```python
from build123d import *

# Parameters (mm, degrees)
SKETCH1_R                = 130.175
SKETCH1_R_2              = 7.874
EXTRUDE1_DEPTH           = 8.89
SKETCH3_R                = 38.1
EXTRUDE3_DEPTH           = 185.309775514
SKETCH4_R                = 5.588
EXTRUDE4_DEPTH           = 185.309775514
EXTRUDE9_DEPTH           = 185.309775514
FILLET1_R                = 7.62
FILLET2_R                = 10.16
CIRPATTERN1_COUNT        = 5
FILLET1_OF_CIRPATTERN1_R = 7.62
FILLET2_OF_CIRPATTERN1_R = 10.16


with BuildPart() as part:
    # Sketch1 → Extrude1 (new body)
    with BuildSketch(Plane.XY):
        Circle(SKETCH1_R)
        with Locations((0, 55)):
            Circle(SKETCH1_R_2, mode=Mode.SUBTRACT)
        with Locations((52.308108396, 16.995934691)):
            Circle(SKETCH1_R_2, mode=Mode.SUBTRACT)
        with Locations((32.328188876, -44.495934691)):
            Circle(SKETCH1_R_2, mode=Mode.SUBTRACT)
        with Locations((-32.328188876, -44.495934691)):
            Circle(SKETCH1_R_2, mode=Mode.SUBTRACT)
        with Locations((-52.308108396, 16.995934691)):
            Circle(SKETCH1_R_2, mode=Mode.SUBTRACT)
    extrude(amount=EXTRUDE1_DEPTH)

    # Sketch3 → Extrude3 (cut, through all)
    with BuildSketch(Plane(origin=(0, 0, 0), x_dir=(-1, 0, 0), z_dir=(0, 0, -1))):
        Circle(SKETCH3_R)
    extrude(amount=-EXTRUDE3_DEPTH, mode=Mode.SUBTRACT)

    # Sketch4 → Extrude4 (cut, through all)
    with BuildSketch(Plane.XY.offset(8.89)):
        with Locations((0, 114.3)):
            Circle(SKETCH4_R)
        with Locations((14.540907903, 100.554074991)):
            Circle(SKETCH4_R)
        with Locations((25.431391759, 85.18482443)):
            Circle(SKETCH4_R)
        with Locations((70.868043945, 72.803024301)):
            Circle(SKETCH4_R)
        with Locations((70.644811643, 53.967773605)):
            Circle(SKETCH4_R)
        with Locations((67.183854337, 92.470642457)):
            Circle(SKETCH4_R)
        with Locations((100.125995916, 17.243692812)):
            Circle(SKETCH4_R)
        with Locations((88.874314608, 2.13686756)):
            Circle(SKETCH4_R)
        with Locations((108.705759813, 35.320642457)):
            Circle(SKETCH4_R)
        with Locations((91.139220605, -44.90214324)):
            Circle(SKETCH4_R)
        with Locations((73.156850119, -50.510249263)):
            Circle(SKETCH4_R)
        with Locations((108.705759813, -35.320642457)):
            Circle(SKETCH4_R)
        with Locations((47.34036073, -89.896886742)):
            Circle(SKETCH4_R)
        with Locations((29.495955395, -83.864167648)):
            Circle(SKETCH4_R)
        with Locations((67.183854337, -92.470642457)):
            Circle(SKETCH4_R)
        with Locations((-14.540907903, -100.554074991)):
            Circle(SKETCH4_R)
        with Locations((-25.431391759, -85.18482443)):
            Circle(SKETCH4_R)
        with Locations((0, -114.3)):
            Circle(SKETCH4_R)
        with Locations((-70.868043945, -72.803024301)):
            Circle(SKETCH4_R)
        with Locations((-70.644811643, -53.967773605)):
            Circle(SKETCH4_R)
        with Locations((-67.183854337, -92.470642457)):
            Circle(SKETCH4_R)
        with Locations((-100.125995916, -17.243692812)):
            Circle(SKETCH4_R)
        with Locations((-88.874314608, -2.13686756)):
            Circle(SKETCH4_R)
        with Locations((-108.705759813, -35.320642457)):
            Circle(SKETCH4_R)
        with Locations((-91.139220605, 44.90214324)):
            Circle(SKETCH4_R)
        with Locations((-73.156850119, 50.510249263)):
            Circle(SKETCH4_R)
        with Locations((-108.705759813, 35.320642457)):
            Circle(SKETCH4_R)
        with Locations((-47.34036073, 89.896886742)):
            Circle(SKETCH4_R)
        with Locations((-29.495955395, 83.864167648)):
            Circle(SKETCH4_R)
        with Locations((-67.183854337, 92.470642457)):
            Circle(SKETCH4_R)
    extrude(amount=-EXTRUDE4_DEPTH, mode=Mode.SUBTRACT)

    # Sketch8 → Extrude9 (cut, through all)
    with BuildSketch(Plane.XY.offset(8.89)):
        Polygon((28.096692809, 71.081575805), (58.920240294, 48.686957693), (31.388364268, 21.595846559), (10.839332611, 36.525591967), align=None)
    extrude9 = extrude(amount=-EXTRUDE9_DEPTH, mode=Mode.SUBTRACT)

    # Fillet1
    fillet1_edges = [part.edges().sort_by_distance(p)[0] for p in [
        (10.839332611, 36.525591967, 4.445),
        (31.388364268, 21.595846559, 4.445),
    ]]
    fillet(fillet1_edges, radius=FILLET1_R)

    # Fillet2
    fillet2_edges = [part.edges().sort_by_distance(p)[0] for p in [
        (28.096692809, 71.081575805, 4.445),
        (58.920240294, 48.686957693, 4.445),
    ]]
    fillet(fillet2_edges, radius=FILLET2_R)

    # CirPattern1: Extrude9 ×5 about axis
    cirpattern1_axis = Axis((0, 0, 0), (0, 0, 1))
    for i in range(1, CIRPATTERN1_COUNT):
        add(extrude9.rotate(cirpattern1_axis, i * 360 / CIRPATTERN1_COUNT), mode=Mode.SUBTRACT)

    # Fillet1 of CirPattern1
    fillet1_of_cirpattern1_edges = [part.edges().sort_by_distance(p)[0] for p in [
        (-31.388364268, 21.595846559, 4.445),
        (-10.839332611, 36.525591967, 4.445),
        (-30.238408579, -23.178624778, 4.445),
        (-38.087440236, 0.978210736, 4.445),
        (12.7, -35.921024484, 4.445),
        (-12.7, -35.921024484, 4.445),
        (38.087440236, 0.978210736, 4.445),
        (30.238408579, -23.178624778, 4.445),
    ]]
    fillet(fillet1_of_cirpattern1_edges, radius=FILLET1_OF_CIRPATTERN1_R)

    # Fillet2 of CirPattern1
    fillet2_of_cirpattern1_edges = [part.edges().sort_by_distance(p)[0] for p in [
        (-58.920240294, 48.686957693, 4.445),
        (-28.096692809, 71.081575805, 4.445),
        (-64.511403936, -40.991381142, 4.445),
        (-76.284951421, -4.756127871, 4.445),
        (19.05, -74.021024484, 4.445),
        (-19.05, -74.021024484, 4.445),
        (76.284951421, -4.756127871, 4.445),
        (64.511403936, -40.991381142, 4.445),
    ]]
    fillet(fillet2_of_cirpattern1_edges, radius=FILLET2_OF_CIRPATTERN1_R)


solid = part.part
```
Work out the finished part from the listing and answer in its coordinate system (mm). Round coordinates to 2 decimals unless told otherwise and drop trailing zeros. Write each loop counter-clockwise with the first axis right and the second up, starting at its lowest first coordinate (ties: lowest second). Pieces come first, ordered by that corner, then holes. Notation, with made-up numbers: (20.5, -36.75) -> (29.5, -36.75) arc R16 cw to (29.5, -6.75) -> close; hole circle Ø7 at (16.5, 62). An arc over 180 degrees is marked (long way). Write each question's results on one line, items separated by ' | '.
1) The part is cut by section B-B (x = -91.5). Write down the section's boundary in (y, z).
Findings:
outline: (-92.59, 0) -> (-7.07, 0) -> (-7.07, 8.89) -> (-92.59, 8.89) -> close; (2.8, 0) -> (39.33, 0) -> (39.33, 8.89) -> (2.8, 8.89) -> close; (50.48, 0) -> (92.59, 0) -> (92.59, 8.89) -> (50.48, 8.89) -> close
2) Flat-ended cylindrical pins translate along their axes: pin 1 (1.5 mm diameter, centred on y = 15.5, z = 2.5, fed in from +X); pin 2 (14.5 mm diameter, centred on x = -100.13, y = -17.24, fed in from -Z); pin 3 (3 mm diameter, centred on y = -38, z = 4.5, fed in from -X); pin 4 (5 mm diameter, centred on x = -82.5, z = 2, fed in from +Y). Find the tip coordinate at first contact, or state that the pin passes through.
Findings:
pin 1: stops at x = 129.34 | pin 2: stops at z = 0 | pin 3: stops at x = -124.95 | pin 4: stops at y = 102.69
3) The part is cut by section D-D (z = 2.75). State how many separate pieces and enclosed holes the cut face has, and give its area (3 significant figures).
Findings:
separate pieces: 1 | enclosed holes: 36 | area: 39,200 mm²
4) The part is cut by section A-A (x = 0). Write down the section's boundary in (y, z) (3 decimals), and give its area (3 significant figures).
Findings:
outline: (-130.175, 0) -> (-119.888, 0) -> (-119.888, 8.89) -> (-130.175, 8.89) -> close; (-108.712, 0) -> (-74.021, 0) -> (-74.021, 8.89) -> (-108.712, 8.89) -> close; (38.1, 0) -> (47.126, 0) -> (47.126, 8.89) -> (38.1, 8.89) -> close; (62.874, 0) -> (108.712, 0) -> (108.712, 8.89) -> (62.874, 8.89) -> close; (119.888, 0) -> (130.175, 0) -> (130.175, 8.89) -> (119.888, 8.89) -> close | area: 979 mm²
5) For a pull along X with two mould halves and no side action, classify faces 1 (the flat face through (27.1, -27.1, 0)), 2 (the cylindrical face through (-0.73, 119.84, 4.51)) as +X half, -X half, draft (parallel to the pull), parting line (faces both ways), or undercut.
Findings:
face 1: draft | face 2: undercut
6) Consider line 1 along X through (y, z) = (-35, 1); line 2 along Y through (x, z) = (95, 1.75); line 3 along Y through (x, z) = (23.5, 2.25). Determine where each line is inside the solid, lowest interval first. Write a range as [from, to].
Findings:
line 1: x = [-125.38, -114.28], [-103.13, -64.04], [-52.98, -15.93], [15.93, 52.98], [64.04, 103.13], [114.28, 125.38] | line 2: y = [-89, -48.94], [-40.86, 15.02], [19.47, 89] | line 3: y = [-128.04, -29.99], [61.63, 79.94], [90.43, 128.04]
7) The part is cut by section C-C (y = -114.3). Write down the section's boundary in (x, z).
Findings:
outline: (-62.3, 0) -> (-5.59, 0) -> (-5.59, 8.89) -> (-62.3, 8.89) -> close; (5.59, 0) -> (62.3, 0) -> (62.3, 8.89) -> (5.59, 8.89) -> close
